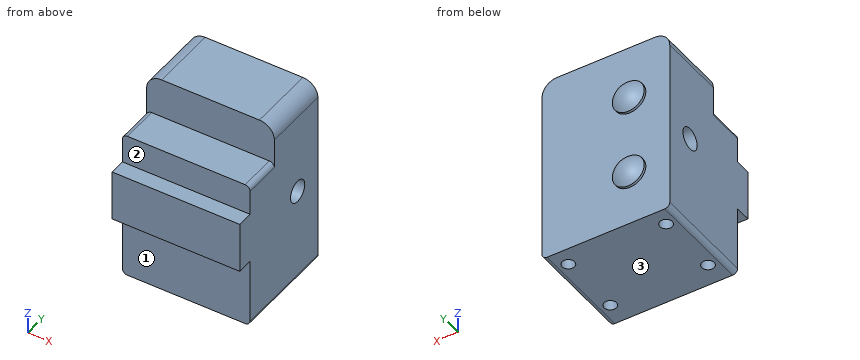
```python
from build123d import *

# Parameters (mm, degrees)
SKETCH1_W           = 25.59
SKETCH1_H           = 38.2
BOSS_EXTRUDE1_DEPTH = 20.97
SKETCH2_W           = 25.59
SKETCH2_H           = 10.2
BOSS_EXTRUDE2_DEPTH = 3.2
SKETCH3_R           = 2.2
CUT_EXTRUDE1_DEPTH  = 25.59
SKETCH4_R           = 1.25
CUT_EXTRUDE2_DEPTH  = 5
FILLET1_R           = 1
FILLET2_R           = 1
FILLET3_R           = 3
SKETCH5_W           = 25.59
SKETCH5_H           = 8
CUT_EXTRUDE3_DEPTH  = 7.5
FILLET4_R           = 1
SKETCH6_R           = 3.2
BOSS_EXTRUDE4_DEPTH = 0.5
DOME1_FACE_RADIUS   = 3.2
DOME1_HEIGHT        = 1.5
DOME2_FACE_RADIUS   = 3.2
DOME2_HEIGHT        = 1.5


with BuildPart() as part:
    # Sketch1 → Boss-Extrude1 (new body)
    with BuildSketch(Plane(origin=(0, 0, 0), x_dir=(1, 0, 0), z_dir=(0, 1, 0))):
        with Locations((12.795, 19.1)):
            Rectangle(SKETCH1_W, SKETCH1_H)
    extrude(amount=BOSS_EXTRUDE1_DEPTH)

    # Sketch2 → Boss-Extrude2 (add)
    with BuildSketch(Plane.XZ):
        with Locations((12.795, -19.1)):
            Rectangle(SKETCH2_W, SKETCH2_H)
    extrude(amount=BOSS_EXTRUDE2_DEPTH)

    # Sketch3 → Cut-Extrude1 (cut)
    with BuildSketch(Plane(origin=(25.59, 0, 0), x_dir=(0, 0, -1), z_dir=(1, 0, 0))):
        with Locations((19.1, 14.7)):
            Circle(SKETCH3_R)
    extrude(amount=-CUT_EXTRUDE1_DEPTH, mode=Mode.SUBTRACT)

    # Sketch4 → Cut-Extrude2 (cut)
    with BuildSketch(Plane(origin=(0, 0, -38.2), x_dir=(-1, 0, 0), z_dir=(0, 0, -1))):
        with Locations((-22.59, 17.47)):
            Circle(SKETCH4_R)
        with Locations((-22.59, 4.5)):
            Circle(SKETCH4_R)
    cut_extrude2 = extrude(amount=-CUT_EXTRUDE2_DEPTH, mode=Mode.SUBTRACT)

    # Fillet1
    fillet1_edges = [part.edges().sort_by_distance(p)[0] for p in [
        (25.59, 10.485, -38.2),
    ]]
    fillet(fillet1_edges, radius=FILLET1_R)

    # Fillet2
    fillet2_edges = [part.edges().sort_by_distance(p)[0] for p in [
        (0, 10.485, -38.2),
    ]]
    fillet(fillet2_edges, radius=FILLET2_R)

    # Fillet3
    fillet3_edges = [part.edges().sort_by_distance(p)[0] for p in [
        (25.59, 10.485, 0),
        (0, 10.485, 0),
    ]]
    fillet(fillet3_edges, radius=FILLET3_R)

    # Sketch5 → Cut-Extrude3 (cut)
    with BuildSketch(Plane.XZ):
        with Locations((12.795, -4)):
            Rectangle(SKETCH5_W, SKETCH5_H)
    extrude(amount=-CUT_EXTRUDE3_DEPTH, mode=Mode.SUBTRACT)

    # Fillet4
    fillet4_edges = [part.edges().sort_by_distance(p)[0] for p in [
        (0, 3.75, -8),
        (25.59, 3.75, -8),
    ]]
    fillet(fillet4_edges, radius=FILLET4_R)

    # Sketch6 → Boss-Extrude4 (add)
    with BuildSketch(Plane(origin=(0, 20.97, 0), x_dir=(1, 0, 0), z_dir=(0, 1, 0))):
        with Locations((8, 27.2)):
            Circle(SKETCH6_R)
    boss_extrude4 = extrude(amount=BOSS_EXTRUDE4_DEPTH)

    # Mirror3: Boss-Extrude4 across plane
    add(boss_extrude4.mirror(Plane(origin=(0, 0, -19.1), x_dir=(1, 0, 0), z_dir=(0, 0, -1))))

    # Dome1: a dome of height H over a round flat face of radius A is a cap of a sphere of radius (A * A + H * H) / (2 * H)
    dome1_r = (DOME1_FACE_RADIUS * DOME1_FACE_RADIUS + DOME1_HEIGHT * DOME1_HEIGHT) / (2 * DOME1_HEIGHT)
    dome1_base = Plane((8, 21.47, -11), z_dir=(0, 1, 0))
    with Locations(dome1_base.offset(DOME1_HEIGHT - dome1_r)):
        dome1_ball = Sphere(dome1_r, mode=Mode.PRIVATE)
    add(split(dome1_ball, bisect_by=dome1_base, keep=Keep.TOP, mode=Mode.PRIVATE))

    # Dome2: a dome of height H over a round flat face of radius A is a cap of a sphere of radius (A * A + H * H) / (2 * H)
    dome2_r = (DOME2_FACE_RADIUS * DOME2_FACE_RADIUS + DOME2_HEIGHT * DOME2_HEIGHT) / (2 * DOME2_HEIGHT)
    dome2_base = Plane((8, 21.47, -27.2), z_dir=(0, 1, 0))
    with Locations(dome2_base.offset(DOME2_HEIGHT - dome2_r)):
        dome2_ball = Sphere(dome2_r, mode=Mode.PRIVATE)
    add(split(dome2_ball, bisect_by=dome2_base, keep=Keep.TOP, mode=Mode.PRIVATE))

    # Mirror4: Cut-Extrude2 across plane
    add(cut_extrude2.mirror(Plane(origin=(12.795, 0, 0), x_dir=(0, 0, 1), z_dir=(1, 0, 0))), mode=Mode.SUBTRACT)


solid = part.part
```
Geometry: final body of the model. Coordinates: model frame, mm. Face numbers are marked on the shaded views. A direction names the side the tool comes from. Coordinates: 2 decimals unless noted, no trailing zeros. Loops run counter-clockwise (first coordinate to the right, second up) from the corner with the lowest first, then second, coordinate; pieces in that order, holes last. Notation, with made-up numbers: (57.25, 42.5) -> (91.25, 42.5) arc R9 cw to (91.25, 46.5) -> close; hole circle Ø6 at (19.5, -10). An arc over 180 degrees is marked (long way). Use a Markdown table: item, result. Add a question column.
(1) Section query C-C, the plane y = 14.7. Return loops of the section in (x, z), plus the area to 3 significant figures.
(2) Section query A-A, the plane z = -19.1. Return loops of the section in (x, y).
(3) Access query for the marked faces 1, 2 and 3. Directions: +Z, -Z, +X, -X, +Y, -Y. A direction counts if a zero-diameter tool reaches every point of the face in a straight line with its end or side. Return the directions, or none.
(4) Section query B-B, the plane x = 19.5. Return loops of the section in (y, z), plus the area to 3 significant figures.
(5) Line query: line 1 along Y through (x, z) = (3, -34.4); line 2 along Y through (x, z) = (4.5, -32); line 3 along Z through (x, y) = (23, -1). Output: solid intervals per line, ascending.
(6) Section query D-D, the plane z = -35. Return loops of the section in (x, y).
(7) Pin query (flat end, axial travel): pin 1 Ø4 at (x, z) = (13, -34) entering from +Y; pin 2 Ø1.8 at (x, z) = (14, -10.5) entering from -Y; pin 3 Ø3 at (x, y) = (22.59, 4.5) entering from -Z; pin 4 Ø4 at (x, y) = (7, 3.5) entering from +Z. Return the tip coordinate at first contact, or that it passes through.
Answer:
| question | item | result |
|---|---|---|
| 1 | outline | (0, -37.2) arc R1 ccw to (1, -38.2) -> (24.59, -38.2) arc R1 ccw to (25.59, -37.2) -> (25.59, -21.3) -> (0, -21.3) -> close; (0, -16.9) -> (25.59, -16.9) -> (25.59, -3) arc R3 ccw to (22.59, 0) -> (3, 0) arc R3 ccw to (0, -3) -> close |
| 1 | area | 861 mm^2 |
| 2 | outline | (0, -3.2) -> (25.59, -3.2) -> (25.59, 12.5) -> (0, 12.5) -> close; (0, 16.9) -> (25.59, 16.9) -> (25.59, 20.97) -> (0, 20.97) -> close |
| 3 | face 1 | -Z, +X, -X, -Y |
| 3 | face 2 | +Z, +X, -X, -Y |
| 3 | face 3 | -Z, +X, -X, +Y, -Y |
| 4 | outline | (-3.2, -24.2) -> (0, -24.2) -> (0, -38.2) -> (20.97, -38.2) -> (20.97, 0) -> (7.5, 0) -> (7.5, -8) -> (0, -8) -> (0, -14) -> (-3.2, -14) -> close; hole circle Ø4.4 at (14.7, -19.1) |
| 4 | area | 758 mm^2 |
| 5 | line 1 | y = 0 to 3.25, 5.75 to 16.22, 18.72 to 20.97 |
| 5 | line 2 | y = 0 to 20.97 |
| 5 | line 3 | z = -24.2 to -14 |
| 6 | outline | (0, 0) -> (25.59, 0) -> (25.59, 20.97) -> (0, 20.97) -> close; hole circle Ø2.5 at (3, 4.5); hole circle Ø2.5 at (3, 17.47); hole circle Ø2.5 at (22.59, 4.5); hole circle Ø2.5 at (22.59, 17.47) |
| 7 | pin 1 | stops at y = 20.97 |
| 7 | pin 2 | stops at y = 0 |
| 7 | pin 3 | stops at z = -38.2 |
| 7 | pin 4 | stops at z = -8 |
